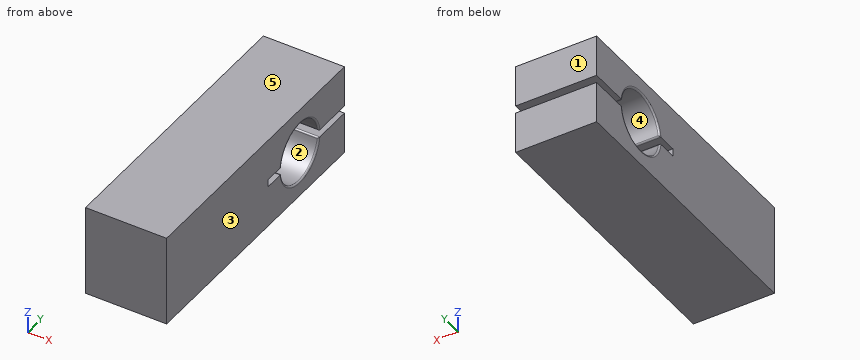
```python
from build123d import *

# Parameters (mm, degrees)
SKETCH1_W           = 25.4
SKETCH1_H           = 28.575
BOSS_EXTRUDE1_DEPTH = 88.9
CUT_EXTRUDE1_REACH  = 98.772
FILLET1_R           = 0.508


with BuildPart() as part:
    # Sketch1 → Boss-Extrude1 (new body)
    with BuildSketch(Plane(origin=(0, 0, 0), x_dir=(1, 0, 0), z_dir=(0, 1, 0))):
        with Locations((12.7, 14.2875)):
            Rectangle(SKETCH1_W, SKETCH1_H)
    extrude(amount=BOSS_EXTRUDE1_DEPTH)

    # Sketch2 → Cut-Extrude1 (cut, up to next)
    with BuildSketch(Plane(origin=(25.4, 0, 0), x_dir=(0, 0, -1), z_dir=(1, 0, 0)), mode=Mode.PRIVATE) as cut_extrude1_sk1:
        with BuildLine():
            Line((13.096875, 50.8), (15.478125, 50.8))
            Line((15.478125, 50.8), (15.478125, 57.224707036))
            ThreePointArc((15.478125, 57.224707036), (23.8125, 66.675), (15.478125, 76.125292964))
            Line((15.478125, 76.125292964), (15.478125, 88.9))
            Line((15.478125, 88.9), (13.096875, 88.9))
            Line((13.096875, 88.9), (13.096875, 76.125292964))
            ThreePointArc((13.096875, 76.125292964), (4.7625, 66.675), (13.096875, 57.224707036))
            Line((13.096875, 57.224707036), (13.096875, 50.8))
        make_face()
    cut_extrude1_tool1 = extrude(cut_extrude1_sk1.sketch, amount=-CUT_EXTRUDE1_REACH, mode=Mode.PRIVATE) & part.part
    add(cut_extrude1_tool1.solids().sort_by_distance((25.4, 67.546559, -14.2875))[0], mode=Mode.SUBTRACT)

    # Fillet1
    fillet1_edges = [part.edges().sort_by_distance(p)[0] for p in [
        (12.7, 57.224707036, -13.096875),
        (12.7, 76.125292964, -13.096875),
        (12.7, 76.125292964, -15.478125),
        (12.7, 57.224707036, -15.478125),
        (25.4, 66.675, -23.8125),
        (25.4, 66.675, -4.7625),
        (0, 66.675, -4.7625),
        (0, 66.675, -23.8125),
    ]]
    fillet(fillet1_edges, radius=FILLET1_R)


solid = part.part
```
Part model, mm, in its own coordinate system. Face numbers are marked on the shaded views. A direction names the side the tool comes from. Coordinates: 2 decimals unless noted, no trailing zeros. Return JSON: item names as keys, results as strings. Group by question number.
Item 1: Pin check, flat tip, straight feed: pin 1 (0.7 mm diameter, centred on x = 14, z = -14.5, fed in from +Y). Stop position of the tip, or through.
Item 2: Drill centre lines: probe 1 along Z at (x, y) = (3.75, 77) (3 decimals); probe 2 along Z at (x, y) = (13, 66.5) (3 decimals); probe 3 along Y at (x, z) = (24, -13.25). Where is each one in solid material? Low to high. Write a range as from..to.
Item 3: Which spindle directions (+Z, -Z, +X, -X, +Y, -Y) get a long thin tool onto all of the face, cutting with end or side? Do the marked faces 4 and 5. Say none if no direction does.
Item 4: Pull direction Y, two halves, no side cores. Call the marked faces 1, 2 and 3: pulls with the +Y half, pulls with the -Y half, needs draft (parallel to the pull), parting line crosses it, or undercut.
Check values:
{
 "1": {"pin 1": "stops at y = 50.8"},
 "2": {"probe 1": "z = -28.575..-15.478, -13.097..0", "probe 2": "z = -28.575..-23.811, -4.764..0", "probe 3": "y = 0..50.8"},
 "3": {"face 4": "+X, -X", "face 5": "+Z, +X, -X, +Y, -Y"},
 "4": {"face 1": "pulls with the +Y half", "face 2": "undercut", "face 3": "needs draft"}
}
